Answer from the drawing. Dimensions are ordinates in mm from the lowest x, y and z of the part. A direction names the side the tool comes from. Give positions to 0.01 mm unless a question says otherwise; leave off trailing zeros. Write each loop counter-clockwise with the first axis right and the second up, starting at its lowest first coordinate (ties: lowest second). Pieces come first, ordered by that corner, then holes.
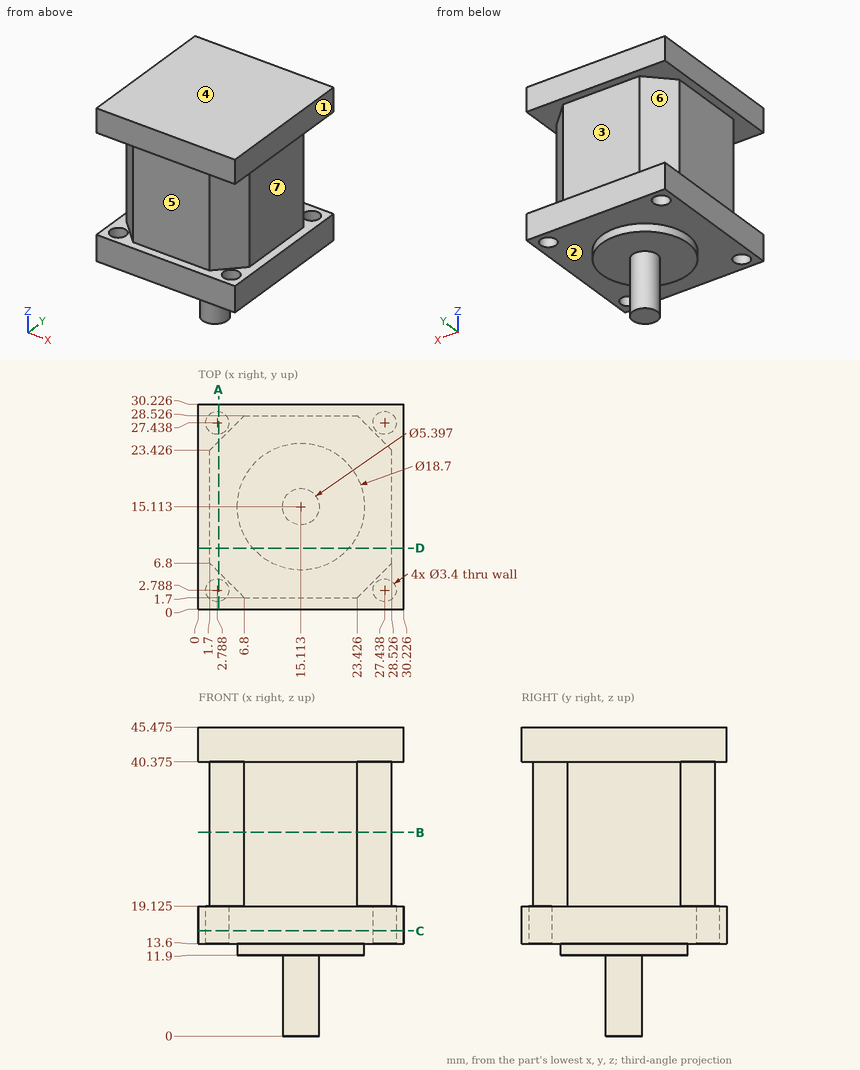
Item 1: Determine the mould class of the marked faces 1, 2, 3 and 4 for opening direction Z: pulls with the +Z half, pulls with the -Z half, needs draft (parallel to the pull), parting line crosses it, or undercut.
Result set:
face 1: needs draft
face 2: pulls with the -Z half
face 3: undercut
face 4: pulls with the +Z half
Item 2: Section C-C (z = 15.5) is taken. Write down the section's boundary in (x, y) (1 decimal), and give its area (3 significant figures).
Result set:
outline: (0, 0) - (30.2, 0) - (30.2, 30.2) - (0, 30.2) - close; hole circle Ø3.4 at (2.8, 2.8); hole circle Ø3.4 at (2.8, 27.4); hole circle Ø3.4 at (27.4, 2.8); hole circle Ø3.4 at (27.4, 27.4)
area: 877 mm2
Item 3: Which of the six approach directions +Z, -Z, +X, -X, +Y, -Y give full straight-line access (tool end or side, diameter ignored) to the marked faces 5, 6 and 7?
Result set:
face 5: +X, -X, -Y
face 6: -X, +Y
face 7: +X, +Y, -Y
Item 4: Find the intervals of material crossed by line 1 along Z through (x, y) = (16, 1) (1 decimal); line 2 along X through (y, z) = (18, 22) (1 decimal), in increasing order.
Result set:
line 1: z = 13.6 to 19.1, 40.4 to 45.5
line 2: x = 1.7 to 28.5
Item 5: Each of these flat-tipped pins is pushed along its axis until it touches: pin 1 Ø2 at (x, y) = (27.438, 2.788) entering from -Z (1 decimal); pin 2 Ø1.5 at (x, y) = (18.5, 9.5) entering from -Z; pin 3 Ø1.5 at (x, z) = (11, 12) entering from -Y; pin 4 Ø10 at (y, z) = (26.5, 13.5) entering from -X. Where does it stop, or does it pass through?
Result set:
pin 1: stops at z = 40.4
pin 2: stops at z = 11.9
pin 3: stops at y = 6.39
pin 4: stops at x = 0
Item 6: Section B-B (z = 30) is taken. Write down the section's boundary in (x, y) (1 decimal), and give its area (3 significant figures).
Result set:
outline: (1.7, 6.8) - (6.8, 1.7) - (23.4, 1.7) - (28.5, 6.8) - (28.5, 23.4) - (23.4, 28.5) - (6.8, 28.5) - (1.7, 23.4) - close
area: 668 mm2
Item 7: Section D-D (y = 9) is taken. Write down the section's boundary in (x, z) (1 decimal), and give its area (3 significant figures).
Result set:
outline: (0, 13.6) - (8, 13.6) - (8, 11.9) - (22.2, 11.9) - (22.2, 13.6) - (30.2, 13.6) - (30.2, 19.1) - (28.5, 19.1) - (28.5, 40.4) - (30.2, 40.4) - (30.2, 45.5) - (0, 45.5) - (0, 40.4) - (1.7, 40.4) - (1.7, 19.1) - (0, 19.1) - close
area: 915 mm2
Item 8: Section A-A (x = 3) is taken. Write down the section's boundary in (y, z) (1 decimal).
Result set:
outline: (0, 13.6) - (1.1, 13.6) - (1.1, 19.1) - (0, 19.1) - close; (0, 40.4) - (5.5, 40.4) - (5.5, 19.1) - (4.5, 19.1) - (4.5, 13.6) - (25.8, 13.6) - (25.8, 19.1) - (24.7, 19.1) - (24.7, 40.4) - (30.2, 40.4) - (30.2, 45.5) - (0, 45.5) - close; (29.1, 13.6) - (30.2, 13.6) - (30.2, 19.1) - (29.1, 19.1) - close
